```python
from build123d import *

# Parameters (mm, degrees)
F0_R     = 23.214461
F1_DEPTH = 25.4


with BuildPart() as f1:
    # F0 (on Top) → F1 (new body)
    with BuildSketch(Plane.XY):
        Polygon((-40.301334, 29.280633), (-40.301334, -29.280633), (15.39374, -47.37706), (49.815189, 0), (15.39374, 47.37706), align=None)
        Circle(F0_R, mode=Mode.SUBTRACT)
    extrude(amount=F1_DEPTH)


solid = f1.part
```
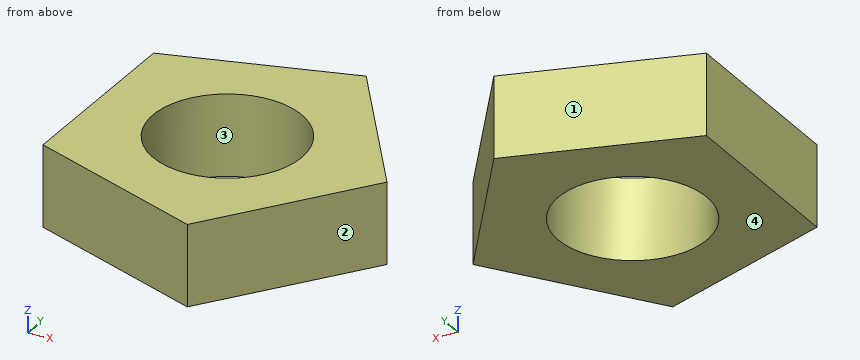
Geometry check sheet. Reference: the model listing, model coordinates, mm. Face numbers are marked on the shaded views. Round coordinates to 2 decimals unless told otherwise and drop trailing zeros. Order: outer loops, then holes, each group sorted by start corner. A loop starts at its lowest first (then second) coordinate and runs counter-clockwise, first axis right, second up. Notation, with made-up numbers: (-11, 50) - (31, 50) arc R30 ccw to (31, 86) - close; hole circle Ø2 at (-3, -29.5). An arc over 180 degrees is marked (long way). Use a Markdown table: item, result. Add a question column.
1) Section check B-B (y = -10). Record the cut outline in (x, z), then the cut area to 3 significant figures.
2) Mould release check, pull along X, two halves, no side actions. Record for the marked faces 1, 2, 3 and 4: released by +X, released by -X, zero draft, split by the parting line, or undercut.
3) Thickness scan on line 1 along Y through (x, z) = (12, 17.75); line 2 along Y through (x, z) = (-11.5, 19.25); line 3 along X through (y, z) = (-13, 18.25). Record the ranges inside material, lowest first.
4) Section check D-D (x = -24.5). Record the cut outline in (y, z), then the cut area to 3 significant figures.
5) Section check C-C (z = 15.5). Record the cut outline in (x, y).
6) Section check A-A (x = -7.5). Record the cut outline in (y, z).
7) Gauge pin test, flat ends, axial feed: P1, Ø2, axis at x = -2, z = 17, coming from the +Y side; P2, Ø3, axis at y = 21.5, z = 13.5, coming from the +X side; P3, Ø1.5, axis at y = -7, z = 17, coming from the +X side. Record the tip position at first contact, or that the pin passes through.
Established:
| question | item | result |
|---|---|---|
| 1 | outline | (-40.3, 0) - (-20.95, 0) - (-20.95, 25.4) - (-40.3, 25.4) - close; (20.95, 0) - (42.55, 0) - (42.55, 25.4) - (20.95, 25.4) - close |
| 1 | area | 1,040 mm2 |
| 2 | face 1 | released by -X |
| 2 | face 2 | released by +X |
| 2 | face 3 | undercut |
| 2 | face 4 | zero draft |
| 3 | line 1 | -46.27 to -19.87, 19.87 to 46.27 |
| 3 | line 2 | -38.64 to -20.17, 20.17 to 38.64 |
| 3 | line 3 | -40.3 to -19.23, 19.23 to 40.37 |
| 4 | outline | (-34.41, 0) - (34.41, 0) - (34.41, 25.4) - (-34.41, 25.4) - close |
| 4 | area | 1,750 mm2 |
| 5 | outline | (-40.3, -29.28) - (15.39, -47.38) - (49.82, 0) - (15.39, 47.38) - (-40.3, 29.28) - close; hole circle Ø46.43 at (0, 0) |
| 6 | outline | (-39.94, 0) - (-21.97, 0) - (-21.97, 25.4) - (-39.94, 25.4) - close; (21.97, 0) - (39.94, 0) - (39.94, 25.4) - (21.97, 25.4) - close |
| 7 | P1 | y = 42.05 |
| 7 | P2 | x = 35.28 |
| 7 | P3 | x = 45.27 |
